Can you work these out from the model? Positions are in its coordinate system, mm. Give positions to 0.01 mm unless a question says otherwise; leave off trailing zeros. Order: outer loops, then holes, each group sorted by start corner. A loop starts at its lowest first (then second) coordinate and runs counter-clockwise, first axis right, second up. Notation, with made-up numbers: M -31,-5.5 L 25,-5.5 A30 ccw 25,33.5 Z; hole C -27,71.25 d10. An arc over 180 degrees is marked long. Write each question's results on one line, items separated by ' | '.
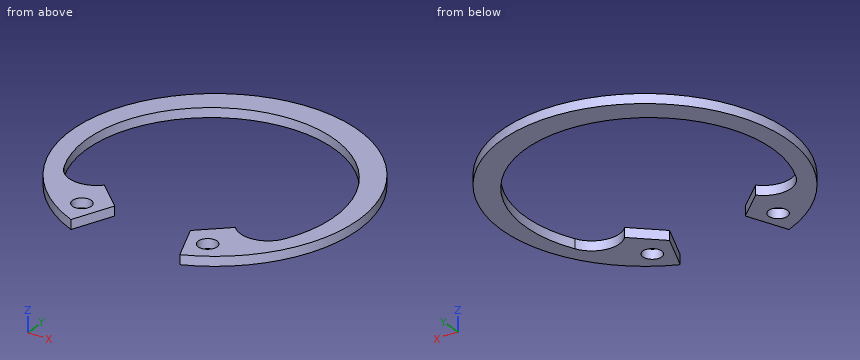
from build123d import *

# Parameters (mm, degrees)
EXTRUDE_1003_DEPTH      = 0.75
EXTRUDE_1003_DEPTH_BACK = 0.75
SKETCH_1_R              = 1.5


with BuildPart() as part:
    # Sketch 1 → Extrude 1003 (new, two sides: drawn at the far end of the back side and taken through both)
    with BuildSketch(Plane.XY.offset(-EXTRUDE_1003_DEPTH_BACK)):
        with BuildLine():
            Line((-10.491561876, -10.592532295), (-6.065532403, -14.64349059))
            Line((-6.065532403, -14.64349059), (-8.706048086, -21.018259365))
            ThreePointArc((-8.706048086, -21.018259365), (0, 22.75), (8.706048086, -21.018259365))
            Line((8.706048086, -21.018259365), (6.065532403, -14.64349059))
            Line((6.065532403, -14.64349059), (10.491561876, -10.592532295))
            ThreePointArc((10.491561876, -10.592532295), (14.377460618, -11.975014118), (17.700870528, -9.532390201))
            ThreePointArc((17.700870528, -9.532390201), (0, 18.65), (-17.700870528, -9.532390201))
            ThreePointArc((-17.700870528, -9.532390201), (-14.377460618, -11.975014118), (-10.491561876, -10.592532295))
        make_face()
        with Locations((-10.067656556, -16.46609521)):
            Circle(SKETCH_1_R, mode=Mode.SUBTRACT)
        with Locations(Location((10.067656556, -16.46609521, 0), (0, 0, 180))):
            Circle(SKETCH_1_R, mode=Mode.SUBTRACT)
    extrude(amount=EXTRUDE_1003_DEPTH + EXTRUDE_1003_DEPTH_BACK)


solid = part.part
(1) Imagine slicing it at D-D, the plane x = 0. Write out the boundary of the cut face in (y, z), plus the area to 3 significant figures.
Data:
outline: M 18.65,-0.75 L 22.75,-0.75 L 22.75,0.75 L 18.65,0.75 Z | area: 6.15 mm2
(2) Imagine slicing it at B-B, the plane y = -1. Write out the boundary of the cut face in (x, z).
Data:
outline: M -22.73,-0.75 L -19.65,-0.75 L -19.65,0.75 L -22.73,0.75 Z; M 19.65,-0.75 L 22.73,-0.75 L 22.73,0.75 L 19.65,0.75 Z
(3) Imagine slicing it at A-A, the plane x = 7.5. Write out the boundary of the cut face in (y, z), plus the area to 3 significant figures.
Data:
outline: M -18.11,-0.75 L -13.33,-0.75 L -13.33,0.75 L -18.11,0.75 Z; M 17.16,-0.75 L 21.48,-0.75 L 21.48,0.75 L 17.16,0.75 Z | area: 13.6 mm2
(4) Imagine slicing it at C-C, the plane z = 0.2. Write out the boundary of the cut face in (x, y), plus the area to 3 significant figures.
Data:
outline: M -17.7,-9.53 A19.65 cw long 17.7,-9.53 A4.4 cw 10.49,-10.59 L 6.07,-14.64 L 8.71,-21.02 A22.75 ccw long -8.71,-21.02 L -6.07,-14.64 L -10.49,-10.59 A4.4 cw Z; hole C -10.07,-16.47 d3; hole C 10.07,-16.47 d3 | area: 450 mm2
(5) I need wall thicknesses on L1, parallel to X at y = -17, z = 0.05; L2, parallel to Y at x = -15.5, z = 0.4; L3, parallel to X at y = 8, z = 0. Which ranges of each line are inside material? Lowest first, please. Write a range as from..to.
Data:
L1: x = -15.12..-11.47, -8.67..-7.04, 7.04..8.67, 11.47..15.12 | L2: y = -16.65..-11.65, 11.08..16.65 | L3: x = -21.3..-17.47, 17.47..21.3
